Here's how the part is built. I have some questions about the finished solid (model axes, mm). Coordinates: 2 decimals unless noted, no trailing zeros. Loops run counter-clockwise (first coordinate to the right, second up) from the corner with the lowest first, then second, coordinate; pieces in that order, holes last. Notation, with made-up numbers: M 29,70.25 L 78,70.25 A9 cw 78,86.25 Z; hole C -18,-11 d3. An arc over 180 degrees is marked long. Use one line per item in the form item = value. Start each with the question number.
(1) Imagine slicing it at C-C, the plane y = 0.5. Please give me the cut outline in (x, z).
(2) Will these pins go through, and if not, where does the flat tip stop? P1, Ø1, axis at y = 1, z = -134.5, coming from the +X side; P2, Ø1, axis at y = 1, z = 63.5, coming from the +X side.
(3) Imagine slicing it at B-B, the plane z = -266.5. Please give me the cut outline in (x, y), and give its area (3 significant figures).
(4) Please list where these lines run through material, in increasing order: L1, parallel to Z at x = -148, y = 1.8; L2, parallel to X at y = 0.75, z = -137.5; L3, parallel to X at y = 0.8, z = 348.
(5) Imagine slicing it at A-A, the plane x = 124. Please give me the cut outline in (y, z).
(6) Thinking about a two-plate mould opening in X: for faces 1 (the flat face through (475.924, 0.986, 229.276)), 2 (the flat face through (449.18, 0.99, 219.18)), 3 (the flat face through (-394, 2, 33)), which applies, +X half, -X half, draft (parallel to the pull), parting line (faces both ways), or undercut?
```python
from build123d import *

# Parameters (mm, degrees)
EXTRUDE_1_DEPTH = 2


with BuildPart() as part:
    # 草图1 → 凸台-拉伸1 (new body)
    with BuildSketch(Plane(origin=(0, 0, 0), x_dir=(1, 0, 0), z_dir=(0, 1, 0))):
        Polygon((-409, 458), (-409, -460), (541, -460), (409, 8), (409, 458), align=None)
        Polygon((386, 435), (-386, 435), (-386, -437), (510.615467151, -437), (386, 4.818474445), align=None, mode=Mode.SUBTRACT)
    extrude(amount=EXTRUDE_1_DEPTH)


solid = part.part
```
Answer:
q1.outline = M -409,-458 L 409,-458 L 409,-8 L 541,460 L -409,460 Z; hole M -386,-435 L 386,-435 L 386,-4.82 L 510.62,437 L -386,437 Z
q2.P1 = 409
q2.P2 = 429.31
q3.outline = M -409,0 L -386,0 L -386,2 L -409,2 Z; M 386,0 L 409,0 L 409,2 L 386,2 Z
q3.area = 92.0 mm²
q4.L1 = -458 to -435, 437 to 460
q4.L2 = -409 to -386, 386 to 409
q4.L3 = -409 to -386, 485.51 to 509.41
q5.outline = M 0,-458 L 2,-458 L 2,-435 L 0,-435 Z; M 0,437 L 2,437 L 2,460 L 0,460 Z
q6.face_1 = +X half
q6.face_2 = undercut
q6.face_3 = draft
